Geometry: see drawing. Coordinates: mm, zero at the bounding-box minimum. A direction names the side the tool comes from. Coordinates: 2 decimals unless noted, no trailing zeros. Order: outer loops, then holes, each group sorted by start corner. A loop starts at its lowest first (then second) coordinate and runs counter-clockwise, first axis right, second up.
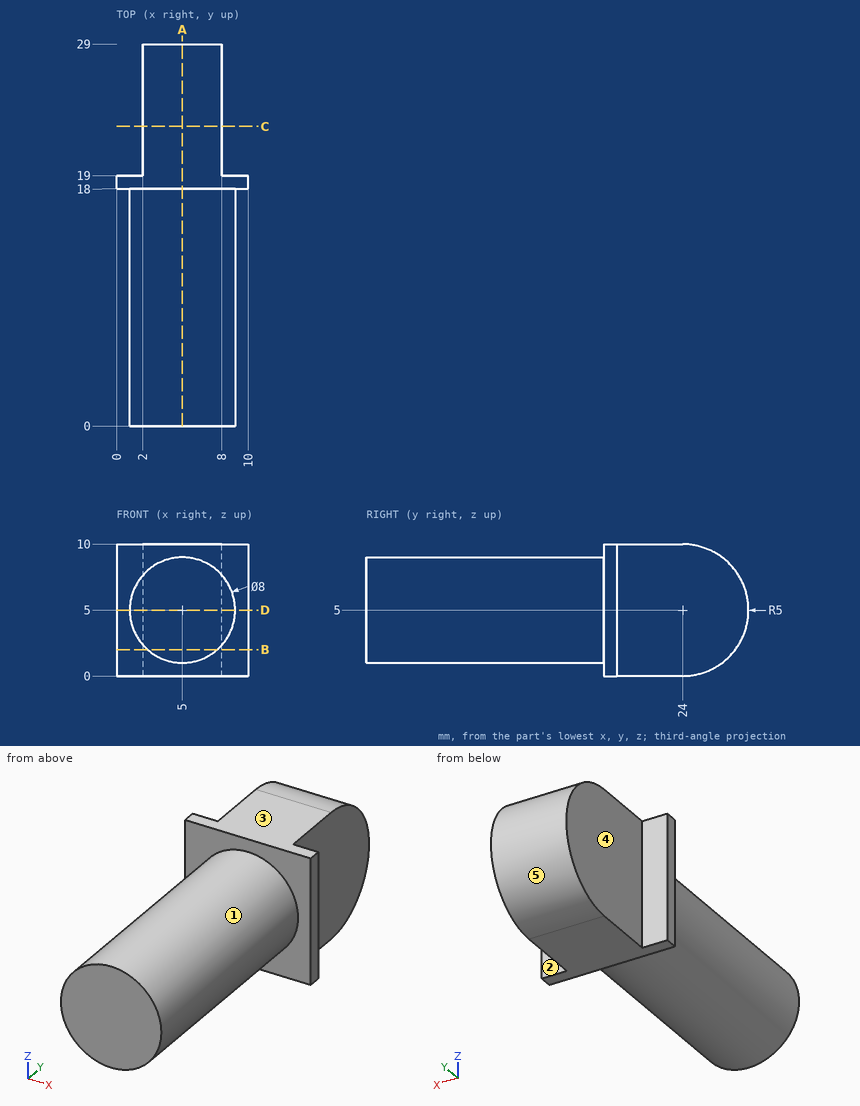
Item 1: Pin query (flat end, axial travel): pin 1 Ø6 at (y, z) = (13, 8) entering from +X; pin 2 Ø5 at (x, z) = (4.5, 3) entering from -Y; pin 3 Ø1 at (x, y) = (8, 7) entering from -Z; pin 4 Ø2 at (y, z) = (7.5, 8) entering from -X. Return the tip coordinate at first contact, or that it passes through.
Response values:
pin 1: stops at x = 9
pin 2: stops at y = 0
pin 3: stops at z = 1.88
pin 4: stops at x = 1.54
Item 2: Cut plane D-D on z = 5. Return loops of the section in (x, y).
Response values:
outline: (0, 18) - (1, 18) - (1, 0) - (9, 0) - (9, 18) - (10, 18) - (10, 19) - (8, 19) - (8, 29) - (2, 29) - (2, 19) - (0, 19) - close
Item 3: Cut plane C-C on y = 22.75. Return loops of the section in (x, z), then the cut area to 3 significant figures.
Response values:
outline: (2, 0) - (8, 0) - (8, 10) - (2, 10) - close
area: 60.0 mm2
Item 4: Ray query, probe 1 along Z at (x, y) = (4.25, 27); probe 2 along Y at (x, z) = (1.75, 4); probe 3 along Y at (x, z) = (8.75, 2). Return the intervals inside material, ascending.
Response values:
probe 1: z = 1 to 9
probe 2: y = 0 to 19
probe 3: y = 18 to 19
Item 5: Cut plane B-B on z = 2. Return loops of the section in (x, y).
Response values:
outline: (0, 18) - (2.35, 18) - (2.35, 0) - (7.65, 0) - (7.65, 18) - (10, 18) - (10, 19) - (8, 19) - (8, 28) - (2, 28) - (2, 19) - (0, 19) - close
Item 6: Access query for the marked faces 1, 2, 3, 4 and 5. Directions: +Z, -Z, +X, -X, +Y, -Y. A direction counts if a zero-diameter tool reaches every point of the face in a straight line with its end or side. Return the directions, or none.
Response values:
face 1: -Y
face 2: +Z, -Z, +X, +Y
face 3: +Z, +X, -X, +Y, -Y
face 4: +Z, -Z, -X, +Y
face 5: +X, -X, +Y
Item 7: Cut plane A-A on x = 5. Return loops of the section in (y, z).
Response values:
outline: (0, 1) - (18, 1) - (18, 0) - (24, 0) arc R5 ccw to (24, 10) - (18, 10) - (18, 9) - (0, 9) - close
